Could you check a few things on this drawing? It's one solid part, dimensions in mm from its lowest x, y, z. Give positions to 0.01 mm unless a question says otherwise; leave off trailing zeros. Loops run counter-clockwise (first coordinate to the right, second up) from the corner with the lowest first, then second, coordinate; pieces in that order, holes last. Notation, with made-up numbers: M 18,-36.75 L 63,-36.75 A25 ccw 63,-7.75 Z; hole C -36.5,5 d3. An arc over 180 degrees is marked long. One line per item, written item: value. Start each with the question number.
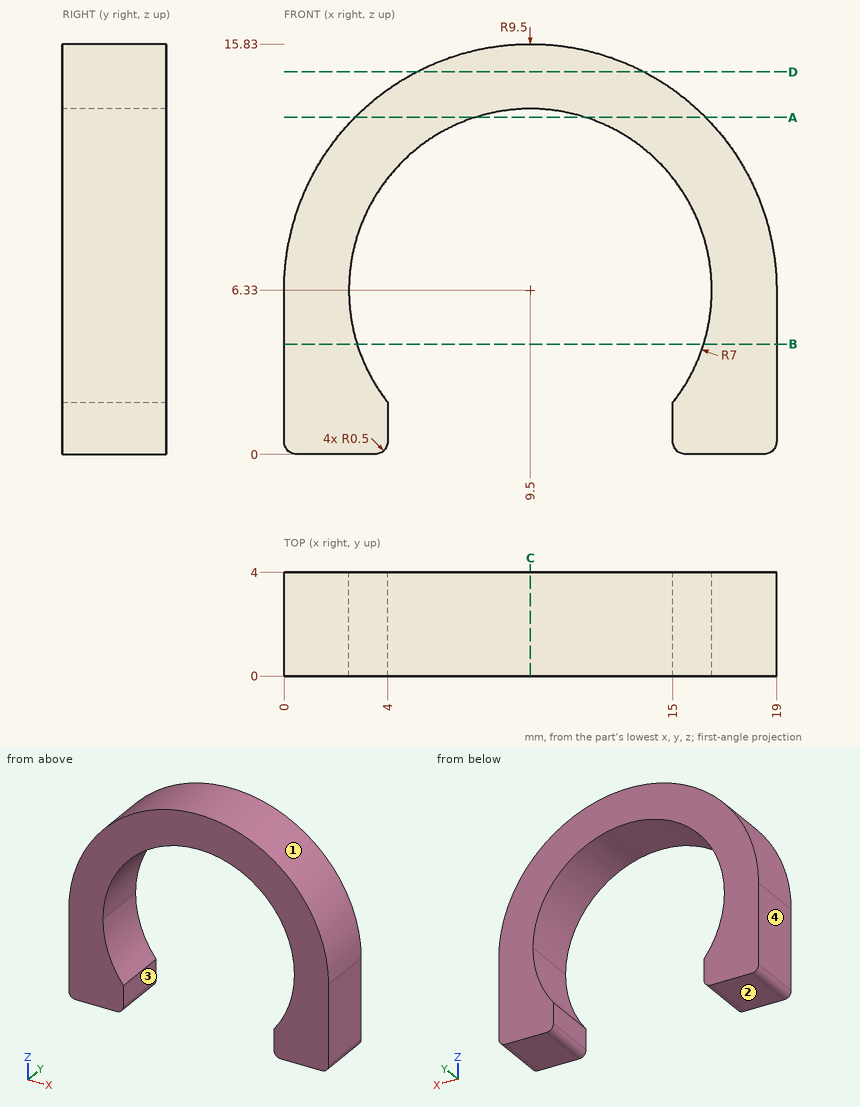
Q1. If we mould it in two halves opening along X, with no side actions, what happens to the marked faces 1, 2, 3 and 4? For each: released by +X, released by -X, zero draft, split by the parting line, or undercut.
Q2. If we section it at D-D, the plane z = 14.75: Write out the boundary of the cut face in (x, y).
Q3. For P1, Ø5, axis at x = 12, z = 12.5, coming from the +Y side; P2, Ø1.5, axis at y = 3, z = 13, coming from the -X side, each with a flat end and sliding along its axis, tell me the tip position at first contact or that it passes through.
Q4. If we section it at C-C, the plane x = 9.5: Write out the boundary of the cut face in (y, z).
Q5. I need wall thicknesses on line 1 along X through (y, z) = (3.75, 1); line 2 along X through (y, z) = (0.75, 11) (1 decimal); line 3 along Z through (x, y) = (9.5, 3.7). Which ranges of each line are inside material? Lowest first, please.
Q6. If we section it at A-A, the plane z = 13: Write out the boundary of the cut face in (x, y) (1 decimal), plus the area to 3 significant figures.
Q7. If we section it at B-B, the plane z = 4.25: Write out the boundary of the cut face in (x, y), plus the area to 3 significant figures.
Response:
1. face 1: split by the parting line
1. face 2: zero draft
1. face 3: undercut
1. face 4: released by -X
2. outline: M 5.1,0 L 13.9,0 L 13.9,4 L 5.1,4 Z
3. P1: y = 4
3. P2: x = 2.07
4. outline: M 0,13.33 L 4,13.33 L 4,15.83 L 0,15.83 Z
5. line 1: 0 to 4, 15 to 19
5. line 2: 1.2 to 4.3, 14.7 to 17.8
5. line 3: 13.33 to 15.83
6. outline: M 2.7,0 L 7.4,0 L 7.4,4 L 2.7,4 Z; M 11.6,0 L 16.3,0 L 16.3,4 L 11.6,4 Z
6. area: 37.1 mm^2
7. outline: M 0,0 L 2.82,0 L 2.82,4 L 0,4 Z; M 16.18,0 L 19,0 L 19,4 L 16.18,4 Z
7. area: 22.5 mm^2
